Verification items for the finished model (mm, model axes). Face numbers are marked on the shaded views. Round coordinates to 2 decimals unless told otherwise and drop trailing zeros. Write each loop counter-clockwise with the first axis right and the second up, starting at its lowest first coordinate (ties: lowest second). Pieces come first, ordered by that corner, then holes. Notation, with made-up numbers: (-10, 56.25) -> (-5, 56.25) arc R21 cw to (-5, 71.25) -> close; hole circle Ø10 at (65, -25.75). An arc over 180 degrees is marked (long way). Answer as a JSON object with one key per item and string values. Group by question number.
(1) Sectioned sample at C-C on x = -13. Record the cut outline in (y, z).
(2) Scan lines: L1, parallel to X at y = 14, z = 5; L2, parallel to X at y = 1.5, z = 26; L3, parallel to X at y = -5, z = 16.5. Record each from-to range of solid material in increasing order. Write a range as from..to.
(3) Gauge pin test, flat ends, axial feed: pin 1 Ø3 at (x, z) = (-7, 18.5) entering from -Y; pin 2 Ø2 at (x, z) = (-7, 14) entering from -Y; pin 3 Ø4 at (y, z) = (7, 8) entering from +X. Record the tip position at first contact, or that the pin passes through.
(4) Draft check along Z on the marked faces 1, 2 and 3. Enter one of: released by +Z, released by -Z, zero draft, split by the parting line, or undercut.
(5) Sectioned sample at A-A on x = -1. Record the cut outline in (y, z).
(6) Sectioned sample at D-D on x = 3.5. Record the cut outline in (y, z), and give its area (3 significant figures).
(7) Sectioned sample at B-B on z = 30.5. Record the cut outline in (x, y) (3 decimals), and give its area (3 significant figures).
Autodesk Inventor part; units mm, degrees
ref_plane "Work Plane3" through (0, 15.875, 0) normal (0, 0.7071, 0.7071) x (-1, 0, 0)
ref_plane "YZ Plane" through (0, 0, 0) normal (1, 0, 0) x (0, 1, 0)
ref_plane "XY Plane" through (0, 0, 0) normal (0, 0, 1) x (1, 0, 0)
sketch "Sketch1" plane through (0, 0, 0) normal (0, 0, 1) x (1, 0, 0)
  circle A0 centre (0, 0) radius 15.875
  dimension "d0" = 31.75
extrude "Extrusion1" add sketch "Sketch1" along normal blind 38.1
ref_plane "Work Plane2" through (0, 15.875, 0) normal (0, 1, 0) x (-1, 0, 0)
sketch "Sketch4" plane through (0, 15.875, 0) normal (0, 1, 0) x (-1, 0, 0)
  circle A0 centre (0, 7.62) radius 1.4605
  point P0 (0, 0)
  dimension "d6" = 2.921
  dimension "d7" = 7.62
sketch "Sketch5" plane through (0, 0, 0) normal (0, 0, -1) x (-1, 0, 0)
  circle A0 centre (0, 0) radius 15.875
  circle A1 centre (0, 8.255) radius 1.4605
  line L0 (0, 15.875) -> (14.2875, 15.875)
  dimension "d8" = 2.921
  dimension "d9" = 7.62
ref_plane "Work Plane3" through (0, 15.875, 0) normal (0, 0.7071, 0.7071) x (-1, 0, 0)
sketch "Sketch6" plane through (0, 15.875, 0) normal (0, 0.7071, 0.7071) x (-1, 0, 0)
  circle A0 centre (0, 3.9683) radius 1.5875
  point P0 (0, 11.2253)
  dimension "d11" = 3.175
extrude "Extrusion2" add sketch "Sketch6" along normal mid plane 25.4
sketch "Sketch7" plane through (0, 4.0887, -6.1742) normal (0, -0.7071, -0.7071) x (-1, 0, 0)
  circle A0 centre (0, 0) radius 1.5875
  circle A1 centre (0, 0) radius 1.5875
  point P0 (0, -7.257)
hole "Hole1" at (-0.0004, 4.0897, -6.1752) direction (0, 0.7071, 0.7071) diameter 3.302 depth 25.4 tip angle 118
properties part number "Aluminum"
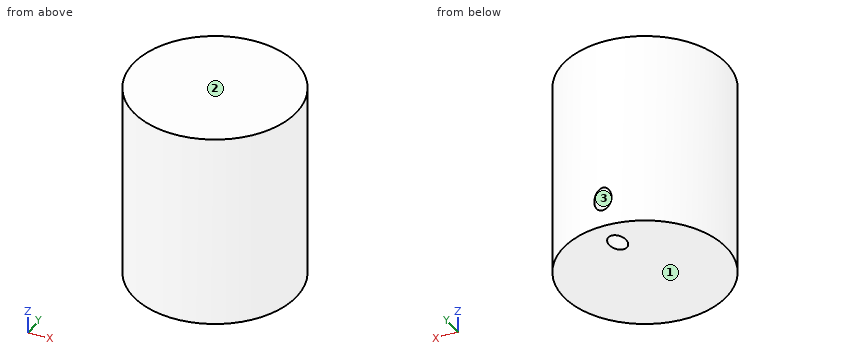
Computed values:
{
 "1": {"outline": "(-9.11, 0) -> (9.11, 0) -> (9.11, 38.1) -> (-9.11, 38.1) -> close"},
 "2": {"L1": "-7.48..-1.39, 1.39..7.48", "L2": "-15.8..15.8", "L3": "-15.07..15.07"},
 "3": {"pin 1": "y = -14.89", "pin 2": "y = -14.7", "pin 3": "x = 15.07"},
 "4": {"face 1": "released by -Z", "face 2": "released by +Z", "face 3": "undercut"},
 "5": {"outline": "(-15.84, 0) -> (8.41, 0) -> (15.84, 7.44) -> (15.84, 38.1) -> (-15.84, 38.1) -> close; (12.12, 0) -> (15.84, 0) -> (15.84, 3.72) -> close"},
 "6": {"outline": "(-15.48, 0) -> (15.48, 0) -> (15.48, 38.1) -> (-15.48, 38.1) -> close", "area": "1,180 mm2"},
 "7": {"outline": "circle Ø31.75 at (0, 0)", "area": "792 mm2"}
}
